The listing builds one solid part. Answer for the finished solid, in the listing's coordinates (mm). Face numbers are marked on the shaded views. A direction names the side the tool comes from. Give positions to 0.01 mm unless a question says otherwise; leave off trailing zeros. Order: outer loops, then holes, each group sorted by start corner. A loop starts at its lowest first (then second) coordinate and runs counter-clockwise, first axis right, second up. Notation, with made-up numbers: (50, 46) - (94, 46) arc R14 ccw to (94, 65) - close; hole circle Ø10 at (20, 8.25). An arc over 180 degrees is marked (long way). Answer in a Markdown table with one row per item. Add a question column.
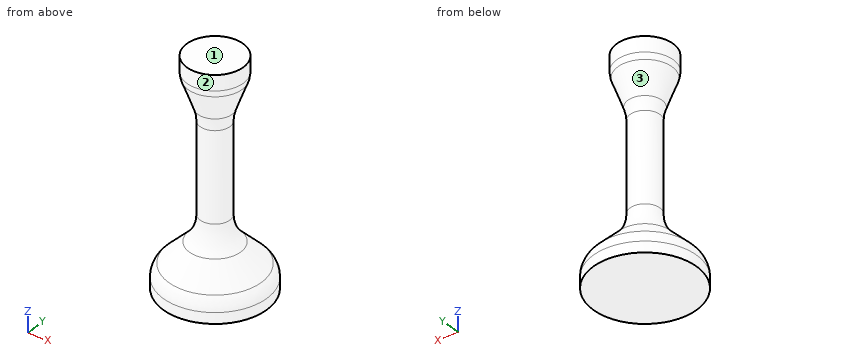
```python
from build123d import *

# Parameters (mm, degrees)
F2_R = 10
F3_R = 5


with BuildPart() as f1:
    # F0 (on Front) → F1 (revolve)
    with BuildSketch(Plane.XZ):
        Polygon((7.6397023427, 30), (0, 30), (0, -30), (7.6397023427, -30), (14, -30), (14, -25), (4, -15), (4, 0), (4, 15), (7.6397023427, 25), align=None)
    revolve(axis=Axis((0, 0, 0), (0, 0, -1)))

    # F2
    f2_edges = [f1.edges().sort_by_distance(p)[0] for p in [
        (-4, 0, 15),
        (-4, 0, -15),
    ]]
    fillet(f2_edges, radius=F2_R)

    # F3
    f3_edges = [f1.edges().sort_by_distance(p)[0] for p in [
        (-7.639702, 0, 25),
        (-14, 0, -25),
    ]]
    fillet(f3_edges, radius=F3_R)


solid = f1.part
```
(1) Each of these flat-tipped pins is pushed along its axis until it touches: P1, Ø5, axis at x = -8.5, y = 10.5, coming from the +Z side; P2, Ø6, axis at x = -0.5, z = 21, coming from the +Y side; P3, Ø1, axis at x = -3, z = 20, coming from the +Y side. Where does it stop, or does it pass through?
(2) For the marked faces 1, 2 and 3, determine the directions among +Z, -Z, +X, -X, +Y, -Y from which every point of the face is accessible in a straight line to the end or side of a thin tool.
(3) Find section B-B, the plane z = 20.5. Write down the section's boundary in (x, y).
(4) Find section A-A, the plane z = 11. Write down the section's boundary in (x, y).
(5) Straight lines are drawn through the part: line 1 (Y direction, x = 0.25, z = -11.5); line 2 (Z direction, x = 9.5, y = 2.75); line 3 (Z direction, x = 5.25, y = 5). For each, find the intervals that lie inside material, in ascending order.
Answer key:
| question | item | result |
|---|---|---|
| 1 | P1 | z = -22.01 |
| 1 | P2 | y = 7.27 |
| 1 | P3 | y = 5.33 |
| 2 | face 1 | +Z, +X, -X, +Y, -Y |
| 2 | face 2 | +Z |
| 2 | face 3 | none |
| 3 | outline | circle Ø12 at (0, 0) |
| 4 | outline | circle Ø8 at (0, 0) |
| 5 | line 1 | -4.01 to 4.01 |
| 5 | line 2 | -30 to -20.89 |
| 5 | line 3 | -30 to -18.25, 23.93 to 30 |
